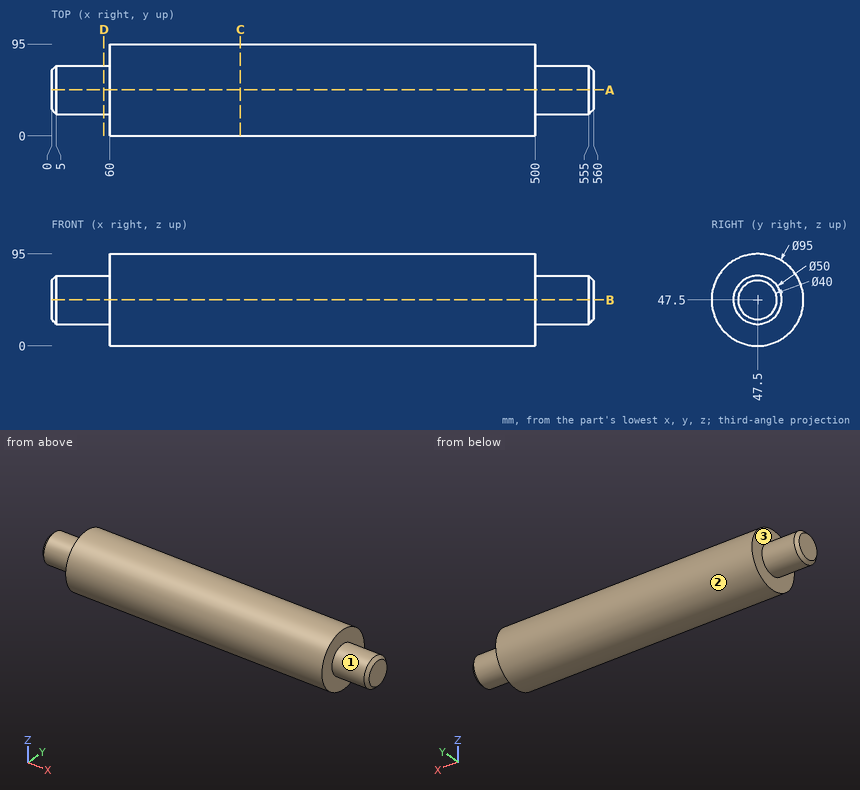
Source: three-view drawing plus pictorial views. Frame: mm from the lowest corner of the part. A direction names the side the tool comes from. Coordinates: 2 decimals unless noted, no trailing zeros. Order: outer loops, then holes, each group sorted by start corner. A loop starts at its lowest first (then second) coordinate and runs counter-clockwise, first axis right, second up.
1) First-contact query: P1, Ø10, axis at y = 67, z = 63.5, coming from the -X side; P2, Ø12, axis at y = 41, z = 43.5, coming from the -X side; P3, Ø12, axis at x = 451, z = 11, coming from the +Y side; P4, Ø1.5, axis at x = 323.5, z = 27, coming from the +Y side. Flat tips, straight axial feed; report the tip coordinate or a pass-through.
Result sheet:
P1: stops at x = 0.22
P2: stops at x = 0
P3: stops at y = 83.91
P4: stops at y = 90.7
2) Section D-D (x = 54). Return loops of the section in (y, z).
Result sheet:
outline: circle Ø50 at (47.5, 47.5)
3) Section C-C (x = 195). Return loops of the section in (y, z).
Result sheet:
outline: circle Ø95 at (47.5, 47.5)
4) Ray query, probe 1 along Y at (x, z) = (205, 46); probe 2 along Z at (x, y) = (48, 48) (3 decimals); probe 3 along X at (y, z) = (68.5, 64). Return the intervals inside material, ascending.
Result sheet:
probe 1: y = 0.02 to 94.98
probe 2: z = 22.505 to 72.495
probe 3: x = 60 to 500
5) Set-up query: the marked faces 1, 2 and 3. Return all of +Z, -Z, +X, -X, +Y, -Y with unobstructed straight access to the full face (end or side cutting, diameter ignored); none if empty.
Result sheet:
face 1: +X
face 2: +X, -X
face 3: -X
6) Section A-A (y = 47.5). Return loops of the section in (x, z), then the cut area to 4 significant figures.
Result sheet:
outline: (0, 27.5) - (5, 22.5) - (60, 22.5) - (60, 0) - (500, 0) - (500, 22.5) - (555, 22.5) - (560, 27.5) - (560, 67.5) - (555, 72.5) - (500, 72.5) - (500, 95) - (60, 95) - (60, 72.5) - (5, 72.5) - (0, 67.5) - close
area: 47,750 mm2
